Build history of the part. All positions in model axes, mm. A direction names the side the tool comes from. Give positions to 0.01 mm unless a question says otherwise; leave off trailing zeros. Loops run counter-clockwise (first coordinate to the right, second up) from the corner with the lowest first, then second, coordinate; pieces in that order, holes last.
1) Band-saw the part on A-A on z = 0. List the corners of the cut face in (x, y), then the cut area to 3 significant figures.
2) Two-plate mould, pull along X, no slides. Class faces 4 (the cylindrical face through (-8, 28, 0)), 5 (the cylindrical face through (-3.905, 14.043, -0.867)), 6 (the flat face through (0, 30.4, 0)): +X half, -X half, draft (parallel to the pull), parting line (faces both ways), or undercut.
3) Wall check: line 1 (X direction, y = 27.6, z = 0); line 2 (Y direction, x = 0, z = 2.45); line 3 (Y direction, x = -13, z = -5.5). Give the ranges that are in metal, low to high.
4) 3-axis set-ups, long thin cutter, end or side, ignore diameter. For faces 1 (the flat face through (0, 3, 2)), 2 (the flat face through (1, 6, 1.6)), 3 (the cylindrical face through (1.25, 4.95, 2.78)): which of +Z, -Z, +X, -X, +Y, -Y reach the whole face in a straight line?
5) Flat gauge pins, fed straight in: P1, Ø5, axis at x = 10, z = 0, coming from the -Y side; P2, Ø12, axis at y = 10, z = 9.5, coming from the +X side; P3, Ø12, axis at x = -14, y = 27.5, coming from the +Z side. Where does each tip first touch, or does it go through?
6) Band-saw the part on B-B on x = 0. List the corners of the cut face in (y, z), then the cut area to 3 significant figures.
7) Band-saw the part on D-D on x = 10. List the corners of the cut face in (y, z).
8) Band-saw the part on C-C on z = -11. List the corners of the cut face in (x, y), then the cut area to 3 significant figures.
```python
from build123d import *

# Parameters (mm, degrees)
CROQUIS1_R              = 4
CROQUIS1_R_2            = 2.05
SALIENTE_EXTRUIR1_DEPTH = 25.4
CROQUIS2_R              = 30
SALIENTE_EXTRUIR2_DEPTH = 5
CROQUIS3_R              = 2
CORTAR_EXTRUIR1_DEPTH   = 7.5
CROQUIS7_R              = 3.5
CORTAR_EXTRUIR3_DEPTH   = 3
CROQUIS8_W              = 62.698346187
CROQUIS8_H              = 3
CORTAR_EXTRUIR5_DEPTH   = 15
CROQUIS1_3_R            = 2.05
CORTAR_EXTRUIR6_DEPTH   = 7.4
SALIENTE_EXTRUIR3_DEPTH = 10
CROQUIS6_R              = 1.25
CORTAR_EXTRUIR7_DEPTH   = 10


with BuildPart() as part:
    # Croquis1 → Saliente-Extruir1 (new body)
    with BuildSketch(Plane(origin=(0, 0, 0), x_dir=(1, 0, 0), z_dir=(0, 1, 0))):
        with Locations(Location((0, 0, 0), (0, 0, 270))):
            Circle(CROQUIS1_R)
        Circle(CROQUIS1_R_2, mode=Mode.SUBTRACT)
        Circle(CROQUIS1_R_2)
    extrude(amount=SALIENTE_EXTRUIR1_DEPTH)

    # Croquis2 → Saliente-Extruir2 (add)
    with BuildSketch(Plane(origin=(0, 25.4, 0), x_dir=(1, 0, 0), z_dir=(0, 1, 0))):
        with Locations(Location((0, 0, 0), (0, 0, 270))):
            Circle(CROQUIS2_R)
    extrude(amount=SALIENTE_EXTRUIR2_DEPTH)

    # Croquis3 → Cortar-Extruir1 (cut)
    with BuildSketch(Plane(origin=(0, 30.4, 0), x_dir=(1, 0, 0), z_dir=(0, 1, 0))):
        with Locations(Location((0, 10, 0), (0, 0, 270))):
            Circle(CROQUIS3_R)
        with Locations(Location((10, 0, 0), (0, 0, 270))):
            Circle(CROQUIS3_R)
        with Locations(Location((0, -10, 0), (0, 0, 270))):
            Circle(CROQUIS3_R)
        with Locations(Location((-10, 0, 0), (0, 0, 270))):
            Circle(CROQUIS3_R)
    extrude(amount=-CORTAR_EXTRUIR1_DEPTH, mode=Mode.SUBTRACT)

    # Croquis7 → Cortar-Extruir3 (cut)
    with BuildSketch(Plane.XZ):
        with Locations(Location((0, 0, 0), (0, 0, 270))):
            Circle(CROQUIS7_R)
    extrude(amount=-CORTAR_EXTRUIR3_DEPTH, mode=Mode.SUBTRACT)

    # Croquis8 → Cortar-Extruir5 (cut, symmetric)
    with BuildSketch(Plane(origin=(0, 0, 0), x_dir=(0, 0, -1), z_dir=(1, 0, 0))):
        with Locations((4.276742622, 1.5)):
            Rectangle(CROQUIS8_W, CROQUIS8_H)
    extrude(amount=CORTAR_EXTRUIR5_DEPTH, both=True, mode=Mode.SUBTRACT)

    # Croquis1<3> → Cortar-Extruir6 (cut)
    with BuildSketch(Plane(origin=(0, 0, 0), x_dir=(1, 0, 0), z_dir=(0, 1, 0))):
        with Locations(Location((0, 0, 0), (0, 0, 90))):
            Circle(CROQUIS1_3_R)
    extrude(amount=CORTAR_EXTRUIR6_DEPTH, mode=Mode.SUBTRACT)

    # Croquis9 → Saliente-Extruir3 (add)
    with BuildSketch(Plane.XZ.offset(-3)):
        with BuildLine():
            ThreePointArc((1.281600562, 1.6), (0, 2.05), (-1.281600562, 1.6))
            Line((-1.281600562, 1.6), (1.281600562, 1.6))
        make_face()
    extrude(amount=-SALIENTE_EXTRUIR3_DEPTH)

    # Croquis6 → Cortar-Extruir7 (cut)
    with BuildSketch(Plane.XY):
        with Locations(Location((0, 5, 0), (0, 0, 180))):
            Circle(CROQUIS6_R)
    extrude(amount=CORTAR_EXTRUIR7_DEPTH, mode=Mode.SUBTRACT)


solid = part.part
```
Findings below:
1. outline: (-30, 25.4) - (-12, 25.4) - (-12, 30.4) - (-30, 30.4) - close; (-8, 25.4) - (-4, 25.4) - (-4, 3) - (-2.05, 3) - (-2.05, 7.4) - (2.05, 7.4) - (2.05, 3) - (4, 3) - (4, 25.4) - (8, 25.4) - (8, 30.4) - (-8, 30.4) - close; (12, 25.4) - (30, 25.4) - (30, 30.4) - (12, 30.4) - close
1. area: 421 mm2
2. face 4: undercut
2. face 5: parting line
2. face 6: draft
3. line 1: x = -30 to -12, -8 to 8, 12 to 30
3. line 2: y = 3 to 3.75, 6.25 to 30.4
3. line 3: y = 25.4 to 30.4
4. face 1: +Z, -Z, +X, -X, -Y
4. face 2: -Y
4. face 3: +Z
5. P1: stops at y = 25.4
5. P2: stops at x = 1.94
5. P3: stops at z = 28.91
6. outline: (3, -4) - (25.4, -4) - (25.4, -8) - (30.4, -8) - (30.4, 8) - (25.4, 8) - (25.4, 4) - (6.25, 4) - (6.25, 1.6) - (7.4, 1.6) - (7.4, -2.05) - (3, -2.05) - close; (3, 1.6) - (3.75, 1.6) - (3.75, 4) - (3, 4) - close; (25.4, -30) - (30.4, -30) - (30.4, -12) - (25.4, -12) - close; (25.4, 12) - (30.4, 12) - (30.4, 30) - (25.4, 30) - close
6. area: 417 mm2
7. outline: (25.4, -28.28) - (30.4, -28.28) - (30.4, -2) - (25.4, -2) - close; (25.4, 2) - (30.4, 2) - (30.4, 28.28) - (25.4, 28.28) - close
8. outline: (-27.91, 25.4) - (-1.73, 25.4) - (-1.73, 30.4) - (-27.91, 30.4) - close; (1.73, 25.4) - (27.91, 25.4) - (27.91, 30.4) - (1.73, 30.4) - close
8. area: 262 mm2
